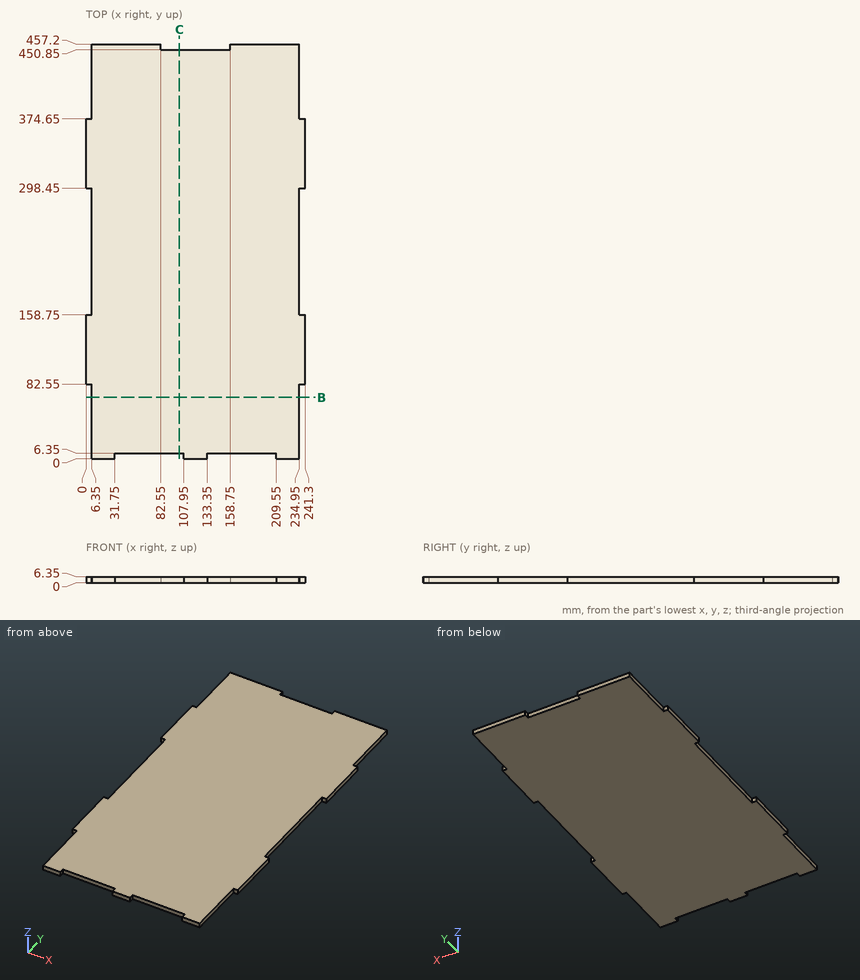
Can you work these out from the drawing? Everything is in mm from the part's minimum corner. Coordinates: 2 decimals unless noted, no trailing zeros. Order: outer loops, then holes, each group sorted by start corner. A loop starts at its lowest first (then second) coordinate and runs counter-clockwise, first axis right, second up. Notation, with made-up numbers: M 66,37.5 L 125,37.5 A13 ccw 125,55.5 Z; hole C -27,-38.75 d10. An arc over 180 degrees is marked long. Answer as CSV lines item,"result". Start each with the question number.
1. I need wall thicknesses on line 1 (Y direction, x = 130.5, z = 3.5); line 2 (Y direction, x = 207.5, z = 4.5); line 3 (X direction, y = 422, z = 5.25). Which ranges of each line are inside material? Lowest first, please. Write a range as [from, to].
2. I want a section at B-B, the plane y = 68. Write out the boundary of the cut face in (x, z), and give its area (3 significant figures).
3. For pin 1 (1.9 mm diameter, centred on x = 2, z = 3.5, fed in from +Y); pin 2 (3 mm diameter, centred on y = 3, z = 2.5, fed in from +X); pin 3 (1.9 mm diameter, centred on y = 233.5, z = 4, fed in from -X), each with a flat end and sliding along its axis, tell me the tip position at first contact or that it passes through.
4. I want a section at C-C, the plane x = 103. Write out the boundary of the cut face in (y, z).
Recorded:
1,line 1,"y = [0, 450.85]"
1,line 2,"y = [6.35, 457.2]"
1,line 3,"x = [6.35, 234.95]"
2,outline,"M 6.35,0 L 234.95,0 L 234.95,6.35 L 6.35,6.35 Z"
2,area,"1,450 mm2"
3,pin 1,"stops at y = 374.65"
3,pin 2,"stops at x = 234.95"
3,pin 3,"stops at x = 6.35"
4,outline,"M 6.35,0 L 450.85,0 L 450.85,6.35 L 6.35,6.35 Z"
